```python
from build123d import *

# Parameters (mm, degrees)
LINK_EYE_SHELF_START      = -23.5
SKETCH1_W                 = 12
SKETCH1_H                 = 12
SKETCH1_R                 = 1.05
LINK_EYE_SHELF_DEPTH      = 2
OUTBOARD_WEB_START        = -22.5
SKETCH2_W                 = 3
SKETCH2_H                 = 12
OUTBOARD_WEB_DEPTH        = 21.5
CARRIAGE_PLATE_FOOT_START = -2
SKETCH3_W                 = 28
SKETCH3_H                 = 12
CARRIAGE_PLATE_FOOT_DEPTH = 2


with BuildPart() as part:
    # Sketch1 → Link_Eye_Shelf (new body)
    with BuildSketch(Plane.XY.offset(LINK_EYE_SHELF_START)):
        with Locations((-38, -20)):
            Rectangle(SKETCH1_W, SKETCH1_H)
        with Locations((-36, -20)):
            Circle(SKETCH1_R, mode=Mode.SUBTRACT)
    extrude(amount=LINK_EYE_SHELF_DEPTH)

    # Sketch2 → Outboard_Web (add)
    with BuildSketch(Plane.XY.offset(OUTBOARD_WEB_START)):
        with Locations((-42.5, -20)):
            Rectangle(SKETCH2_W, SKETCH2_H)
    extrude(amount=OUTBOARD_WEB_DEPTH)

    # Sketch3 → Carriage_Plate_Foot (add)
    with BuildSketch(Plane.XY.offset(CARRIAGE_PLATE_FOOT_START)):
        with Locations((-30, -20)):
            Rectangle(SKETCH3_W, SKETCH3_H)
    extrude(amount=CARRIAGE_PLATE_FOOT_DEPTH)


solid = part.part
```
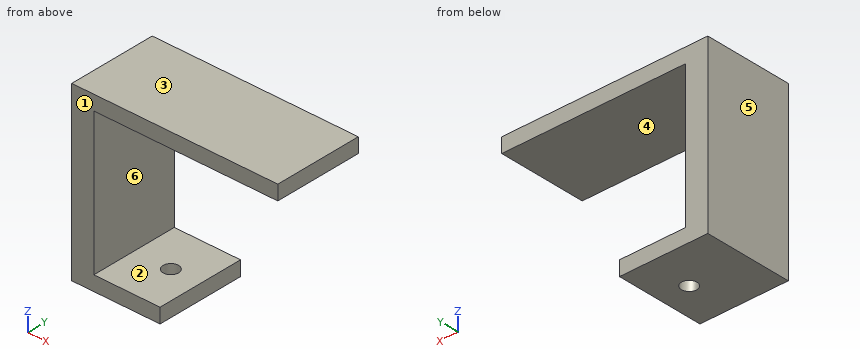
Geometry: final body of the model. Coordinates: model frame, mm. Face numbers are marked on the shaded views. A direction names the side the tool comes from. Coordinates: 2 decimals unless noted, no trailing zeros. Order: outer loops, then holes, each group sorted by start corner. A loop starts at its lowest first (then second) coordinate and runs counter-clockwise, first axis right, second up. Notation, with made-up numbers: (1, 12) -> (42, 12) arc R17 ccw to (42, 23) -> close; hole circle Ø9 at (41, 73). An arc over 180 degrees is marked (long way). Answer in a Markdown table with one row per item.
Item 1: Draft query along Z for the marked faces 1, 2, 3 and 4. Return one class per face: released by +Z, released by -Z, zero draft, split by the parting line, or undercut.
Return value:
| item | result |
|---|---|
| face 1 | zero draft |
| face 2 | undercut |
| face 3 | released by +Z |
| face 4 | undercut |
Item 2: Section D-D on z = -19.5. Output: boundary loops of the cut face in (x, y).
Return value:
| item | result |
|---|---|
| outline | (-44, -26) -> (-41, -26) -> (-41, -14) -> (-44, -14) -> close |
Item 3: Section C-C on y = -16.5. Output: boundary loops of the cut face in (x, z), plus the area to 4 significant figures.
Return value:
| item | result |
|---|---|
| outline | (-44, -23.5) -> (-32, -23.5) -> (-32, -21.5) -> (-41, -21.5) -> (-41, -2) -> (-16, -2) -> (-16, 0) -> (-44, 0) -> close |
| area | 138.5 mm² |
Item 4: Section A-A on y = -20. Output: boundary loops of the cut face in (x, z), plus the area to 3 significant figures.
Return value:
| item | result |
|---|---|
| outline | (-44, -23.5) -> (-37.05, -23.5) -> (-37.05, -21.5) -> (-41, -21.5) -> (-41, -2) -> (-16, -2) -> (-16, 0) -> (-44, 0) -> close; (-34.95, -23.5) -> (-32, -23.5) -> (-32, -21.5) -> (-34.95, -21.5) -> close |
| area | 134 mm² |
Item 5: Section B-B on x = -36. Output: boundary loops of the cut face in (y, z).
Return value:
| item | result |
|---|---|
| outline | (-26, -23.5) -> (-21.05, -23.5) -> (-21.05, -21.5) -> (-26, -21.5) -> close; (-26, -2) -> (-14, -2) -> (-14, 0) -> (-26, 0) -> close; (-18.95, -23.5) -> (-14, -23.5) -> (-14, -21.5) -> (-18.95, -21.5) -> close |
Item 6: Access query for the marked faces 5 and 6. Directions: +Z, -Z, +X, -X, +Y, -Y. A direction counts if a zero-diameter tool reaches every point of the face in a straight line with its end or side. Return the directions, or none.
Return value:
| item | result |
|---|---|
| face 5 | +Z, -Z, -X, +Y, -Y |
| face 6 | +X, +Y, -Y |
Item 7: Contact query for flat-ended pins moving along their axis: P1, Ø1.6, axis at y = -22, z = -22.5, coming from the +X side; P2, Ø5, axis at y = -23.5, z = -10, coming from the +X side; P3, Ø2, axis at x = -28, z = -2.5, coming from the -Y side. Output: stop coordinate, or through.
Return value:
| item | result |
|---|---|
| P1 | stops at x = -32 |
| P2 | stops at x = -41 |
| P3 | stops at y = -26 |
Item 8: Ray query, L1, parallel to Y at x = -36, z = -22.25; L2, parallel to Z at x = -35.5, y = -21.5; L3, parallel to X at y = -25, z = -10. Return the intervals inside material, ascending.
Return value:
| item | result |
|---|---|
| L1 | y = -26 to -21.05, -18.95 to -14 |
| L2 | z = -23.5 to -21.5, -2 to 0 |
| L3 | x = -44 to -41 |
